from build123d import *

# Parameters (mm, degrees)
SKETCH_1_R          = 1.75
EXTRUDE_1_DEPTH     = 3
SKETCH_2_W          = 49.355771561
SKETCH_2_H          = 3.2
CUT_EXTRUDE_1_DEPTH = 1.4


with BuildPart() as part:
    # Эскиз1 → Бобышка-Вытянуть1 (new body)
    with BuildSketch(Plane(origin=(0, 0, 0), x_dir=(1, 0, 0), z_dir=(0, 1, 0))):
        with BuildLine():
            Line((-24.459773103, 5.517931082), (24.895998458, 5.517931082))
            Line((24.895998458, 5.517931082), (24.895998458, -0.482068918))
            Line((24.895998458, -0.482068918), (21.895998458, -0.482068918))
            ThreePointArc((21.895998458, -0.482068918), (15.895998458, -6.482068918), (9.895998458, -0.482068918))
            Line((9.895998458, -0.482068918), (-9.459773103, -0.482068918))
            ThreePointArc((-9.459773103, -0.482068918), (-15.459773103, -6.482068918), (-21.459773103, -0.482068918))
            Line((-21.459773103, -0.482068918), (-24.459773103, -0.482068918))
            Line((-24.459773103, -0.482068918), (-24.459773103, 5.517931082))
        make_face()
        with Locations((15.895998458, -0.482068918)):
            Circle(SKETCH_1_R, mode=Mode.SUBTRACT)
        with Locations((-15.459773103, -0.482068918)):
            Circle(SKETCH_1_R, mode=Mode.SUBTRACT)
    extrude(amount=EXTRUDE_1_DEPTH)

    # Эскиз2 → Вырез-Вытянуть1 (cut)
    with BuildSketch(Plane(origin=(0, 3, 0), x_dir=(1, 0, 0), z_dir=(0, 1, 0))):
        with Locations((0.218112678, 3.917931082)):
            Rectangle(SKETCH_2_W, SKETCH_2_H)
    extrude(amount=-CUT_EXTRUDE_1_DEPTH, mode=Mode.SUBTRACT)


solid = part.part
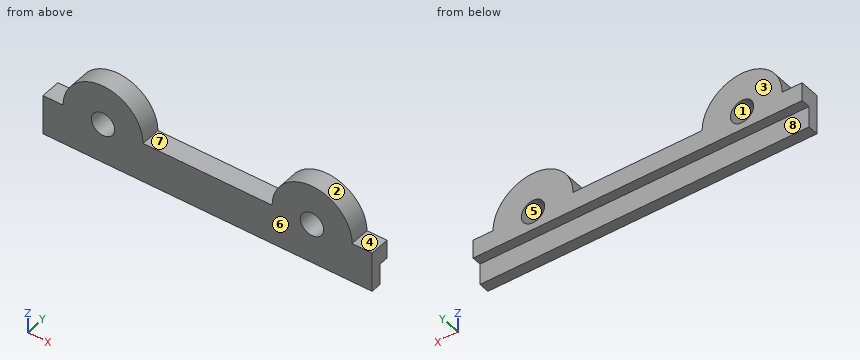
Geometry: final body of the model. Coordinates: model frame, mm. Face numbers are marked on the shaded views. A direction names the side the tool comes from. Round coordinates to 2 decimals unless told otherwise and drop trailing zeros. Loops run counter-clockwise (first coordinate to the right, second up) from the corner with the lowest first, then second, coordinate; pieces in that order, holes last. Notation, with made-up numbers: (45, 82.25) -> (103, 82.25) arc R24 ccw to (103, 108.25) -> close; hole circle Ø11 at (-3, -33.5). An arc over 180 degrees is marked (long way). One line per question, with ' | ' between items. Start each with the question number.
1. Section A-A on y = 2.25. Output: boundary loops of the cut face in (x, z), and give its area (3 significant figures).
2. Section D-D on x = 5. Output: boundary loops of the cut face in (y, z), and give its area (3 significant figures).
3. Section B-B on x = -15. Output: boundary loops of the cut face in (y, z), and give its area (3 significant figures).
4. Set-up query: the marked faces 4, 5, 6, 7 and 8. Return all of +Z, -Z, +X, -X, +Y, -Y with unobstructed straight access to the full face (end or side cutting, diameter ignored); none if empty.
5. Mould query, pull axis Z, two halves, no side actions, for the marked faces 1, 2 and 3. Classes: pulls with the +Z half, pulls with the -Z half, needs draft (parallel to the pull), parting line crosses it, or undercut.
6. Line query: line 1 along X through (y, z) = (2.35, 0.25); line 2 along Y through (x, z) = (-14, -2.5); line 3 along Z through (x, y) = (3, 0.45). Output: solid intervals per line, ascending. Write a range as [from, to].
7. Contact query for flat-ended pins moving along their axis: pin 1 (0.9 mm diameter, centred on x = -23.5, y = 2, fed in from +Z); pin 2 (6 mm diameter, centred on x = -13, z = 3, fed in from -Y); pin 3 (1.1 mm diameter, centred on x = 5.5, y = 2.5, fed in from -Z); pin 4 (1 mm diameter, centred on x = 1, z = -3, fed in from +Y). Output: stop coordinate, or through.
8. Section C-C on z = 3. Output: boundary loops of the cut face in (x, y), and give its area (3 significant figures).
Returned:
1) outline: (-24.46, -2.32) -> (24.9, -2.32) -> (24.9, 0.48) -> (21.9, 0.48) arc R6 ccw to (9.9, 0.48) -> (-9.46, 0.48) arc R6 ccw to (-21.46, 0.48) -> (-24.46, 0.48) -> close; hole circle Ø3.5 at (-15.46, 0.48); hole circle Ø3.5 at (15.9, 0.48) | area: 232 mm2
2) outline: (0, -5.52) -> (1.6, -5.52) -> (1.6, -2.32) -> (3, -2.32) -> (3, 0.48) -> (0, 0.48) -> close | area: 13.5 mm2
3) outline: (0, -5.52) -> (1.6, -5.52) -> (1.6, -2.32) -> (3, -2.32) -> (3, -1.21) -> (0, -1.21) -> close; (0, 2.17) -> (3, 2.17) -> (3, 6.46) -> (0, 6.46) -> close | area: 21.3 mm2
4) face 4: +Z, +X, +Y, -Y | face 5: +Y, -Y | face 6: +Z, -Z, +X, -X, -Y | face 7: +Z, +Y, -Y | face 8: -Z, +X, -X, +Y
5) face 1: undercut | face 2: pulls with the +Z half | face 3: needs draft
6) line 1: x = [-24.46, -17.19], [-13.73, 14.16], [17.63, 24.9] | line 2: y = [0, 1.6] | line 3: z = [-5.52, 0.48]
7) pin 1: stops at z = 0.48 | pin 2: stops at y = 0 | pin 3: stops at z = -2.32 | pin 4: stops at y = 1.6
8) outline: (-20.91, 0) -> (-10.01, 0) -> (-10.01, 3) -> (-20.91, 3) -> close; (10.45, 0) -> (21.34, 0) -> (21.34, 3) -> (10.45, 3) -> close | area: 65.4 mm2
